Can you work these out from the model? Positions are in its coordinate system, mm. Round coordinates to 2 decimals unless told otherwise and drop trailing zeros. Write each loop counter-clockwise with the first axis right and the second up, starting at its lowest first coordinate (ties: lowest second). Pieces come first, ordered by that corner, then holes. Notation, with made-up numbers: (-15, 42.25) -> (-4, 42.25) arc R18 cw to (-4, 52.25) -> close; hole circle Ø4 at (-21.5, 14.5). An arc over 180 degrees is marked (long way). Write item = value, one per line. Start each with the question number.
1) Imagine slicing it at D-D, the plane y = 0.55. State how many separate pieces and enclosed holes the cut face has, then the cut area to 3 significant figures.
2) If I drill on line 1 (X direction, y = 1.2, z = -17.5); line 2 (X direction, y = 1.25, z = 13.75); line 3 (Z direction, x = -11, y = 1.4), over which ranges is the centre line in solid material (lowest first)?
3) Thinking about a two-plate mould opening in Z: for faces 1 (the face through (-32.75, 0.84, -18.04)), 2 (the face through (-1, 0, -7)), which applies, +Z half, -Z half, draft (parallel to the pull), parting line (faces both ways), or undercut?
4) Imagine slicing it at C-C, the plane x = -40. Please give me the cut outline in (y, z).
5) I'm going to push a flat-ended pin straight in: pin 1 (4.5 mm diameter, centred on x = 30.31, z = 17.5, fed in from +Y). Where does the tip first touch, or does it pass through?
6) Imagine slicing it at A-A, the plane x = 0. Please give me the cut outline in (y, z).
7) Imagine slicing it at B-B, the plane z = 35. Please give me the cut outline in (x, y).
from build123d import *

# Parameters (mm, degrees)
SKETCH1_R           = 65
SKETCH1_R_2         = 2.5
SKETCH1_R_3         = 14
SKETCH1_R_4         = 8
BOSS_EXTRUDE1_DEPTH = 1.7


with BuildPart() as part:
    # Sketch1 → Boss-Extrude1 (new body)
    # profile 1 of 2: a face of its own
    with BuildSketch(Plane(origin=(0, 0, 0), x_dir=(1, 0, 0), z_dir=(0, 1, 0))):
        Circle(SKETCH1_R)
        with Locations(Location((-10, 13.75, 0), (0, 0, 270))):
            Circle(SKETCH1_R_2, mode=Mode.SUBTRACT)
        with Locations(Location((10, 13.75, 0), (0, 0, 270))):
            Circle(SKETCH1_R_2, mode=Mode.SUBTRACT)
        with Locations(Location((10, -13.75, 0), (0, 0, 270))):
            Circle(SKETCH1_R_2, mode=Mode.SUBTRACT)
        with Locations(Location((-10, -13.75, 0), (0, 0, 270))):
            Circle(SKETCH1_R_2, mode=Mode.SUBTRACT)
        with Locations(Location((0, 35, 0), (0, 0, 270))):
            Circle(SKETCH1_R_2, mode=Mode.SUBTRACT)
        with Locations(Location((30.310889132, 17.5, 0), (0, 0, 270))):
            Circle(SKETCH1_R_2, mode=Mode.SUBTRACT)
        with Locations(Location((30.310889132, -17.5, 0), (0, 0, 270))):
            Circle(SKETCH1_R_2, mode=Mode.SUBTRACT)
        with Locations(Location((0, -35, 0), (0, 0, 270))):
            Circle(SKETCH1_R_2, mode=Mode.SUBTRACT)
        with Locations(Location((-30.310889132, -17.5, 0), (0, 0, 270))):
            Circle(SKETCH1_R_2, mode=Mode.SUBTRACT)
        with Locations(Location((-30.310889132, 17.5, 0), (0, 0, 270))):
            Circle(SKETCH1_R_2, mode=Mode.SUBTRACT)
    # profile 2 of 2: a face of its own
    with BuildSketch(Plane(origin=(0, 0, 0), x_dir=(1, 0, 0), z_dir=(0, 1, 0))):
        with Locations((-40, 63.718686589)):
            Circle(SKETCH1_R_3)
        with Locations(Location((-40, 63.718686589, 0), (0, 0, 270))):
            Circle(SKETCH1_R_4, mode=Mode.SUBTRACT)
    extrude(amount=BOSS_EXTRUDE1_DEPTH)


solid = part.part
Reported:
q1.separate_pieces = 1
q1.enclosed_holes = 11
q1.area = 13,400 mm²
q2.line_1 = -62.6 to -32.81, -27.81 to 27.81, 32.81 to 62.6
q2.line_2 = -63.53 to -12.5, -7.5 to 7.5, 12.5 to 63.53
q2.line_3 = -64.06 to -16.04, -11.46 to 11.46, 16.04 to 64.06
q3.face_1 = undercut
q3.face_2 = draft
q4.outline = (0, -77.72) -> (1.7, -77.72) -> (1.7, -71.72) -> (0, -71.72) -> close; (0, -55.72) -> (1.7, -55.72) -> (1.7, 51.23) -> (0, 51.23) -> close
q5.pin_1 = through
q6.outline = (0, -65) -> (1.7, -65) -> (1.7, -37.5) -> (0, -37.5) -> close; (0, -32.5) -> (1.7, -32.5) -> (1.7, 32.5) -> (0, 32.5) -> close; (0, 37.5) -> (1.7, 37.5) -> (1.7, 65) -> (0, 65) -> close
q7.outline = (-54.77, 0) -> (-2.5, 0) -> (-2.5, 1.7) -> (-54.77, 1.7) -> close; (2.5, 0) -> (54.77, 0) -> (54.77, 1.7) -> (2.5, 1.7) -> close
